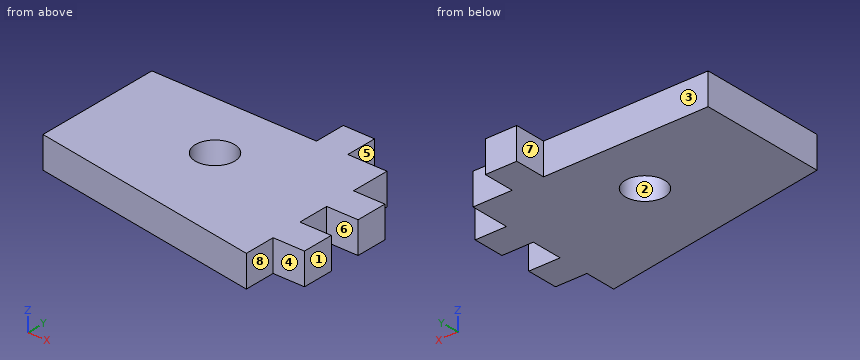
```python
from build123d import *

# Parameters (mm, degrees)
SKETCH1_R           = 2.5
BOSS_EXTRUDE1_DEPTH = 4
SKETCH2_W           = 4
SKETCH2_H           = 4
BOSS_EXTRUDE2_DEPTH = 4


with BuildPart() as part:
    # Sketch1 → Boss-Extrude1 (new body)
    with BuildSketch(Plane.XY):
        Polygon((0, 9.539473684), (0, -11.460526316), (-30, -6.708993106), (-30, 9.539473684), align=None)
        with Locations((-15, 1.415240289)):
            Circle(SKETCH1_R, mode=Mode.SUBTRACT)
    extrude(amount=BOSS_EXTRUDE1_DEPTH)

    # Sketch2 → Boss-Extrude2 (add)
    with BuildSketch(Plane.XY.offset(4)):
        with Locations((2, 2.539473684)):
            Rectangle(SKETCH2_W, SKETCH2_H)
        with Locations((-7, 11.539473684)):
            Rectangle(SKETCH2_W, SKETCH2_H)
        with Locations((2, -5.460526316)):
            Rectangle(SKETCH2_W, SKETCH2_H)
    extrude(amount=-BOSS_EXTRUDE2_DEPTH)


solid = part.part
```
Check sheet for the modelled part. Datum: model origin and axes. Units: mm. Face numbers are marked on the shaded views. A direction names the side the tool comes from. Coordinates: 2 decimals unless noted, no trailing zeros. Loops run counter-clockwise (first coordinate to the right, second up) from the corner with the lowest first, then second, coordinate; pieces in that order, holes last.
1) Gauge pin test, flat ends, axial feed: pin 1 (1.2 mm diameter, centred on x = -2.5, z = 1.5, fed in from +Y); pin 2 (2 mm diameter, centred on x = 1.5, z = 1, fed in from -Y); pin 3 (2 mm diameter, centred on y = -0.5, z = 1.5, fed in from +X); pin 4 (4.5 mm diameter, centred on x = -15, y = 1.42, fed in from -Z). Record the tip position at first contact, or that the pin passes through.
2) Sectioned sample at C-C (z = 0.5). Record the boundary of the cut face in (x, y), and give its area (3 significant figures).
3) Access from +Z, -Z, +X, -X, +Y, -Y to the whole of each face (thin tool, end or side, straight path). Record for the marked faces 5, 6, 7 and 8.
4) Sectioned sample at B-B (x = -15). Record the boundary of the cut face in (y, z).
5) Sectioned sample at A-A (y = 1). Record the boundary of the cut face in (x, z), and give its area (3 significant figures).
6) Sectioned sample at D-D (y = 7). Record the boundary of the cut face in (x, z).
7) Release check for a two-part mould opening along Y. For the marked faces 1, 2, 3 and 4 record: released by +Y, released by -Y, zero draft, split by the parting line, or undercut.
8) Material ranges on probe 1 along X at (y, z) = (1.5, 1.9); probe 2 along Y at (x, z) = (-13.5, 2.3); probe 3 along X at (y, z) = (2.75, 0.8), recorded low to high.
Check sheet entries:
1. pin 1: stops at y = 9.54
1. pin 2: stops at y = -7.46
1. pin 3: stops at x = 0
1. pin 4: passes through
2. outline: (-30, -6.71) - (0, -11.46) - (0, -7.46) - (4, -7.46) - (4, -3.46) - (0, -3.46) - (0, 0.54) - (4, 0.54) - (4, 4.54) - (0, 4.54) - (0, 9.54) - (-5, 9.54) - (-5, 13.54) - (-9, 13.54) - (-9, 9.54) - (-30, 9.54) - close; hole circle Ø5 at (-15, 1.42)
2. area: 587 mm2
3. face 5: +Z, -Z, +X, +Y
3. face 6: +Z, -Z, +X
3. face 7: +Z, -Z, -X, +Y
3. face 8: +Z, -Z, +X, -Y
4. outline: (-9.08, 0) - (-1.08, 0) - (-1.08, 4) - (-9.08, 4) - close; (3.92, 0) - (9.54, 0) - (9.54, 4) - (3.92, 4) - close
5. outline: (-30, 0) - (-17.47, 0) - (-17.47, 4) - (-30, 4) - close; (-12.53, 0) - (4, 0) - (4, 4) - (-12.53, 4) - close
5. area: 116 mm2
6. outline: (-30, 0) - (0, 0) - (0, 4) - (-30, 4) - close
7. face 1: zero draft
7. face 2: undercut
7. face 3: released by +Y
7. face 4: released by -Y
8. probe 1: x = -30 to -17.5, -12.5 to 4
8. probe 2: y = -9.32 to -0.58, 3.42 to 9.54
8. probe 3: x = -30 to -17.11, -12.89 to 4
